```python
from build123d import *


with BuildPart() as part:
    # Austragung4: sweep along a path in Skizze1
    with BuildLine(Plane.XY) as austragung4_path:
        Line((0, 0), (0, 86))
        ThreePointArc((0, 86), (1.7573593128807152, 90.24264068711929), (6, 92.00000000000001))
        Line((6, 92.00000000000001), (16, 92))
    # Skizze3 → Austragung4 (sweep)
    with BuildSketch(Plane(origin=(0, 0, 0), x_dir=(1, 0, 0), z_dir=(0, 1, 0))):
        Polygon((-0.5773502691896251, 1), (-1.1547005383792512, -1.7e-16), (-0.577350269189625, -1.0000000000000009), (0.5773502691896264, -1.0000000000000007), (1.1547005383792524, -2.9e-16), (0.5773502691896265, 1), align=None)
    sweep(path=austragung4_path.line)

    # Skizze6 → Rotation5 (revolve)
    with BuildSketch(Plane(origin=(0, 0, 0), x_dir=(0, 0, -1), z_dir=(1, 0, 0))):
        with BuildLine():
            Line((1.08e-15, -1.0000000000000007), (1.08e-15, 1.0000000000000007))
            ThreePointArc((1.08e-15, 1.0000000000000007), (1.0000000000000007, 0), (1.08e-15, -1.0000000000000007))
        make_face()
    revolve(axis=Axis((0, 7.810357944094903, -1.48e-15), (0, -1, 0)))

    # Skizze8 → Schnitt-Rotation1 (revolve, cut)
    with BuildSketch(Plane.XY, mode=Mode.PRIVATE) as schnitt_rotation1_sk:
        with BuildLine():
            Line((-3.0586465116527903, -0.25356146909949984), (-1.1547005383792512, 0))
            ThreePointArc((-1.1547005383792512, 0), (-0.33900397376978075, 0.6461318381885482), (-0.9758944689717856, 1.469064238181372))
            Line((-0.9758944689717856, 1.469064238181372), (-3.0586465116527903, 1.7464385309005002))
            Line((-3.0586465116527903, 1.7464385309005002), (-3.0586465116527903, -0.25356146909949984))
        make_face()
    revolve(schnitt_rotation1_sk.sketch.rotate(Axis((0, 0, 0), (0, 1, 0)), 270), axis=Axis((0, 0, 0), (0, 1, 0)), mode=Mode.SUBTRACT)


solid = part.part
```
Read the model definition and answer for the solid it produces. Units are mm, in the model's axes. Round coordinates to 2 decimals unless told otherwise and drop trailing zeros. Write each loop counter-clockwise with the first axis right and the second up, starting at its lowest first coordinate (ties: lowest second). Pieces come first, ordered by that corner, then holes. Notation, with made-up numbers: (85, 67.5) - (128, 67.5) arc R23 cw to (128, 98.5) - close; hole circle Ø10 at (18, 78.5). An arc over 180 degrees is marked (long way). One line per item, written item: value.
Q1. Find section B-B (x = 11). Determine the outline of the cut face in (y, z).
The answers:
outline: (90.85, 0) - (91.42, -1) - (92.58, -1) - (93.15, 0) - (92.58, 1) - (91.42, 1) - close
Q2. Straight lines are drawn through the part: line 1 (X direction, y = 86, z = 0.3); line 2 (Y direction, x = 9.5, z = 0); line 3 (Y direction, x = 5, z = 0.2). For each, find the intervals that lie inside material, in ascending order. Write a range as from..to.
The answers:
line 1: x = -0.98..0.98
line 2: y = 90.85..93.15
line 3: y = 90.86..92.97
Q3. Find section A-A (y = 14). Determine the outline of the cut face in (x, z).
The answers:
outline: (-1.15, 0) - (-0.58, -1) - (0.58, -1) - (1.15, 0) - (0.58, 1) - (-0.58, 1) - close
